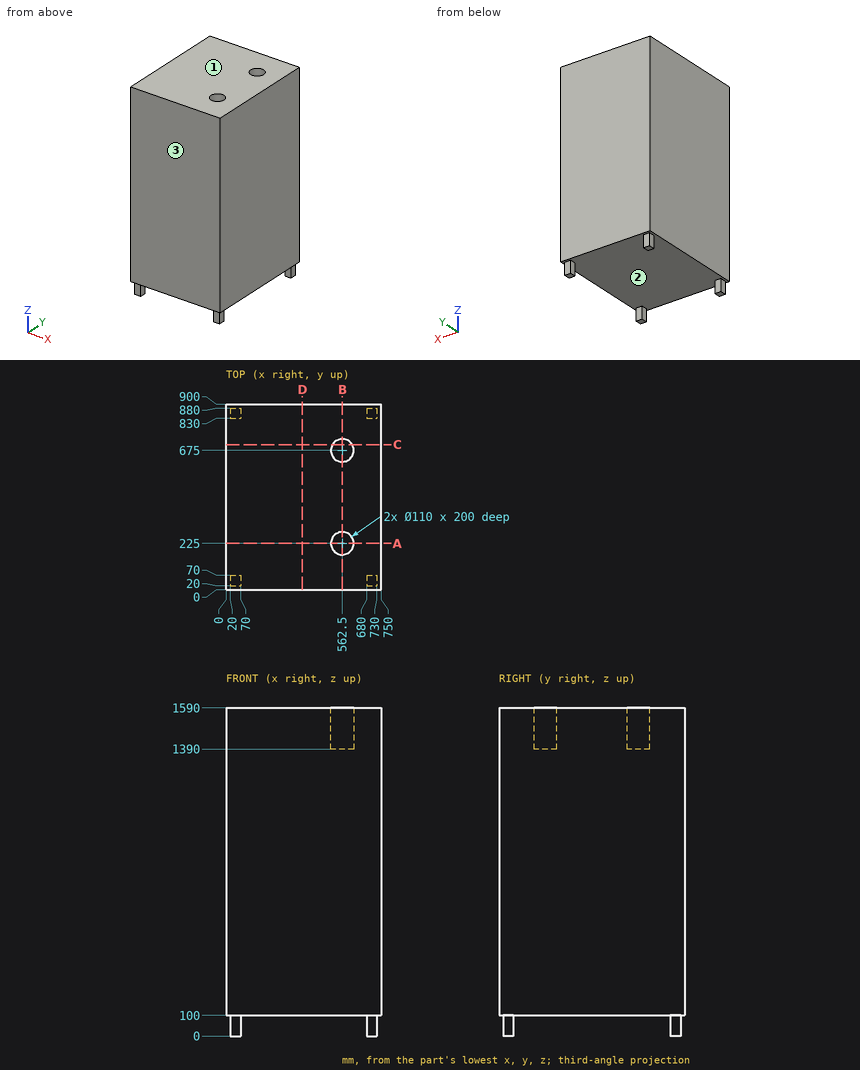
Check sheet for the drawn part. Datum: minimum x, y, z corner. Units: mm. Round coordinates to 2 decimals unless told otherwise and drop trailing zeros. Loops run counter-clockwise (first coordinate to the right, second up) from the corner with the lowest first, then second, coordinate; pieces in that order, holes last. Notation, with made-up numbers: M -33.5,46 L -3.5,46 A10 cw -3.5,60 Z; hole C 5,5 d8. An arc over 180 degrees is marked long. Write each question's results on one line, items separated by ' | '.
1) Section check A-A on y = 225. Record the boundary of the cut face in (x, z).
Checks:
outline: M 0,100 L 750,100 L 750,1590 L 617.5,1590 L 617.5,1390 L 507.5,1390 L 507.5,1590 L 0,1590 Z
2) Mould release check, pull along Y, two halves, no side actions. Record for the marked faces 1, 2 and 3: released by +Y, released by -Y, zero draft, split by the parting line, or undercut.
Checks:
face 1: zero draft | face 2: undercut | face 3: released by -Y
3) Section check D-D on x = 369. Record the boundary of the cut face in (y, z), then the cut area to 3 significant figures.
Checks:
outline: M 0,100 L 900,100 L 900,1590 L 0,1590 Z | area: 1,340,000 mm2
4) Scan lines: L1, parallel to Y at x = 562, z = 1445; L2, parallel to Z at x = 501, y = 580.5; L3, parallel to Z at x = 566.5, y = 223.5. Record each from-to range of solid material in increasing order. Write a range as from..to.
Checks:
L1: y = 0..170, 280..620, 730..900 | L2: z = 100..1590 | L3: z = 100..1390
5) Gauge pin test, flat ends, axial feed: P1, Ø15, axis at y = 864.5, z = 48, coming from the -X side; P2, Ø6, axis at x = 212.5, y = 364.5, coming from the -Z side; P3, Ø15, axis at x = 700.5, z = 45.5, coming from the +Y side; P4, Ø10, axis at y = 114, z = 686.5, coming from the -X side. Record the tip position at first contact, or that the pin passes through.
Checks:
P1: stops at x = 20 | P2: stops at z = 100 | P3: stops at y = 880 | P4: stops at x = 0
6) Section check B-B on x = 562.5. Record the boundary of the cut face in (y, z), then the cut area to 3 significant figures.
Checks:
outline: M 0,100 L 900,100 L 900,1590 L 730,1590 L 730,1390 L 620,1390 L 620,1590 L 280,1590 L 280,1390 L 170,1390 L 170,1590 L 0,1590 Z | area: 1,300,000 mm2
7) Section check C-C on y = 703.5. Record the boundary of the cut face in (x, z), then the cut area to 3 significant figures.
Checks:
outline: M 0,100 L 750,100 L 750,1590 L 609.54,1590 L 609.54,1390 L 515.46,1390 L 515.46,1590 L 0,1590 Z | area: 1,100,000 mm2
